Read the model definition and answer for the solid it produces. Units are mm, in the model's axes. Face numbers are marked on the shaded views. Give positions to 0.01 mm unless a question says otherwise; leave off trailing zeros. Loops run counter-clockwise (first coordinate to the right, second up) from the corner with the lowest first, then second, coordinate; pieces in that order, holes last. Notation, with made-up numbers: (-7, -23) -> (37, -23) arc R17 ccw to (37, 2) -> close; hole circle Ø1 at (67, 10.25). An arc over 180 degrees is marked (long way). Return JSON: item names as keys, results as strings. Group by question number.
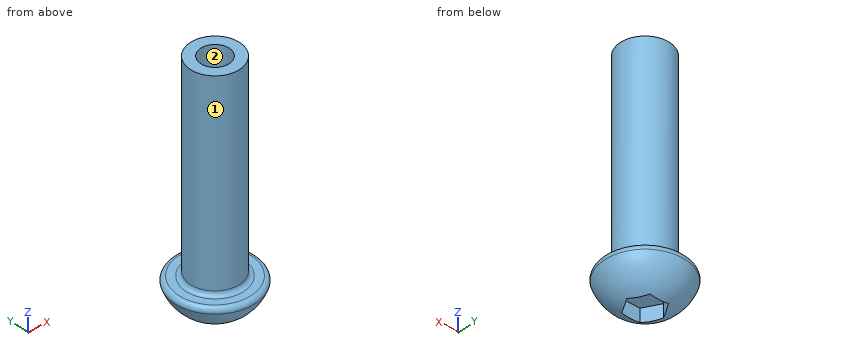
Autodesk Inventor part; units mm, degrees
ref_plane "Work Plane1" through (0, 0, -5.3975) normal (0, 0, 1) x (1, 0, 0)
ref_plane "YZ Plane" through (0, 0, 0) normal (1, 0, 0) x (0, 1, 0)
ref_plane "XZ Plane" through (0, 0, 0) normal (0, 1, 0) x (-1, 0, 0)
sketch "Sketch1" plane through (0, 0, 0) normal (0, 0, 1) x (1, 0, 0)
  circle A0 centre (0, 0) radius 1.8733
  dimension "d0" = 3.7465
extrude "Extrusion1" add sketch "Sketch1" along normal blind 15.24
sketch "Sketch2" plane through (0, 0, 0) normal (0, 0, -1) x (-1, 0, 0)
  circle A0 centre (0, 0) radius 1.8732
  circle A1 centre (0, 0) radius 3.175
  dimension "d3" = 6.35
extrude "Extrusion2" add sketch "Sketch2" along normal blind 2.54 contours A0 | A1
fillet "Fillet1" radius 3.175 1 edges at (3.175, 0, -2.54)
fillet "Fillet2" radius 0.3175 1 edges at (3.175, 0, 0)
fillet "Fillet3" radius 0.3175 1 edges at (-1.8733, 0, 0)
ref_plane "Work Plane1" through (0, 0, -5.3975) normal (0, 0, 1) x (1, 0, 0)
sketch "Sketch4" plane through (0, 0, -5.3975) normal (0, 0, 1) x (1, 0, 0)
  line L0 (1.3748, 0) -> (0.6874, -1.1906)
  line L1 (0.6874, -1.1906) -> (-0.6874, -1.1906)
  line L2 (-0.6874, -1.1906) -> (-1.3748, 0)
  line L3 (-1.3748, 0) -> (-0.6874, 1.1906)
  line L4 (-0.6874, 1.1906) -> (0.6874, 1.1906)
  line L5 (0.6874, 1.1906) -> (1.3748, 0)
  point P0 (0, 0)
  point P1 (0, 0)
  dimension "d19" = 2.3813
extrude "Extrusion3" cut sketch "Sketch4" along normal blind 4.1275
sketch "Sketch5" plane through (0, 0, 15.24) normal (0, 0, 1) x (1, 0, 0)
  point P0 (0, 0)
hole "Hole1" at (0, 0, 15.24) direction (0, 0, -1) diameter 2.159 depth 5.6896 tip angle 118
properties part number "Axel - Female" material "PBT Plastic"
1. Straight lines are drawn through the part: line 1 (Y direction, x = 0, z = 12.95); line 2 (Y direction, x = 0.5, z = 13.75); line 3 (Z direction, x = 0.75, y = -2). For each, find the intervals that lie inside material, in ascending order. Write a range as from..to.
2. Section A-A on z = 12 is taken. Determine the outline of the cut face in (x, y), then the cut area to 3 significant figures.
3. Flat-ended cylindrical pins translate along their axes: pin 1 Ø3 at (x, y) = (0, 0) entering from +Z; pin 2 Ø3 at (x, z) = (-1.5, 9) entering from +Y; pin 3 Ø3 at (x, z) = (2.5, 0.5) entering from -Y; pin 4 Ø1 at (y, z) = (0, 6) entering from -X. Find the tip coordinate at first contact, or state that the pin passes through.
4. Section B-B on z = 5.75 is taken. Determine the outline of the cut face in (x, y).
5. Determine the mould class of the marked faces 1 and 2 for opening direction X: pulls with the +X half, pulls with the -X half, needs draft (parallel to the pull), parting line crosses it, or undercut.
Completed:
{
 "1": {"line 1": "y = -1.87..-1.08, 1.08..1.87", "line 2": "y = -1.81..-0.96, 0.96..1.81", "line 3": "z = -1.77..0"},
 "2": {"outline": "circle Ø3.75 at (0, 0); hole circle Ø2.16 at (0, 0)", "area": "7.36 mm²"},
 "3": {"pin 1": "stops at z = 15.24", "pin 2": "stops at y = 1.87", "pin 3": "stops at y = -2.82", "pin 4": "stops at x = -1.87"},
 "4": {"outline": "circle Ø3.75 at (0, 0)"},
 "5": {"face 1": "parting line crosses it", "face 2": "undercut"}
}
